Study the drawing (mm; zero at the part's minimum x, y, z) and answer. Round coordinates to 2 decimals unless told otherwise and drop trailing zeros. Loops run counter-clockwise (first coordinate to the right, second up) from the corner with the lowest first, then second, coordinate; pieces in that order, holes last. Notation, with made-up numbers: (88.5, 63) - (112.5, 63) arc R27 cw to (112.5, 89) - close; hole circle Ø3 at (35.25, -31.5). An arc over 180 degrees is marked (long way). One line per item, written item: value.
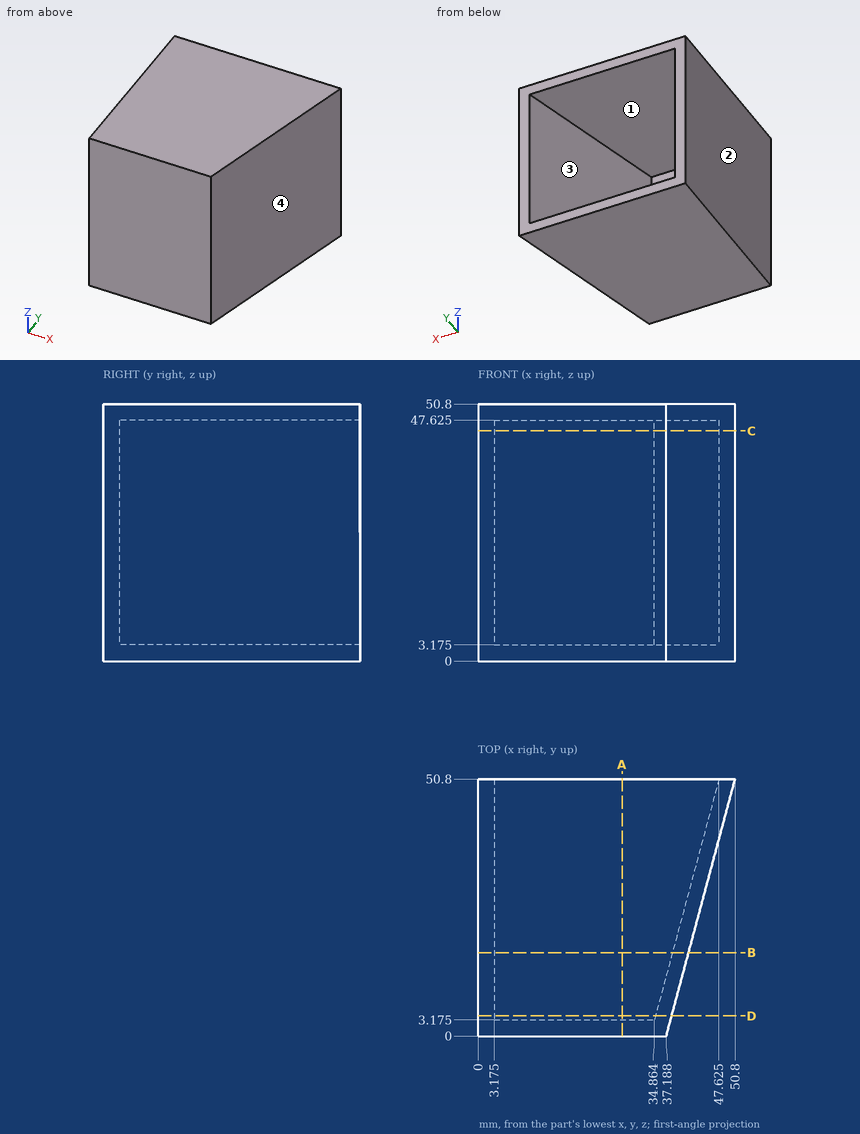
1) Consider L1, parallel to Z at x = 13.5, y = 14.5 (3 decimals); L2, parallel to Y at x = 8, z = 41.5 (3 decimals); L3, parallel to X at y = 43.5, z = 8.5 (1 decimal). Determine where each line is inside the solid, lowest interval first.
Final values:
L1: 0 to 3.175, 47.625 to 50.8
L2: 0 to 3.175
L3: 0 to 3.2, 45.7 to 48.8
2) A cutting plane is placed at A-A on x = 28.5. Give the vertices of the cut face in (y, z) (3 decimals).
Final values:
outline: (0, 0) - (50.8, 0) - (50.8, 3.175) - (3.175, 3.175) - (3.175, 47.625) - (50.8, 47.625) - (50.8, 50.8) - (0, 50.8) - close
3) A cutting plane is placed at D-D on y = 4. Give the vertices of the cut face in (x, z) (3 decimals).
Final values:
outline: (0, 0) - (38.26, 0) - (38.26, 50.8) - (0, 50.8) - close; hole (3.175, 3.175) - (35.085, 3.175) - (35.085, 47.625) - (3.175, 47.625) - close
4) A cutting plane is placed at B-B on y = 16.5. Give the vertices of the cut face in (x, z) (1 decimal).
Final values:
outline: (0, 0) - (41.6, 0) - (41.6, 50.8) - (0, 50.8) - close; hole (3.2, 3.2) - (38.4, 3.2) - (38.4, 47.6) - (3.2, 47.6) - close
5) For a pull along X with two mould halves and no side action, classify the marked faces 1, 2, 3 and 4 as released by +X, released by -X, zero draft, split by the parting line, or undercut.
Final values:
face 1: undercut
face 2: released by -X
face 3: undercut
face 4: released by +X
6) Each of these flat-tipped pins is pushed along its axis until it touches: pin 1 Ø22 at (y, z) = (30.5, 20.5) entering from +X; pin 2 Ø8 at (y, z) = (28, 12.5) entering from +X; pin 3 Ø2 at (x, z) = (7.5, 26.5) entering from +Y (3 decimals). Where does it stop, or does it pass through?
Final values:
pin 1: x = 48.31
pin 2: x = 45.76
pin 3: y = 3.175
7) A cutting plane is placed at C-C on z = 45.5. Give the vertices of the cut face in (x, y) (1 decimal).
Final values:
outline: (0, 0) - (37.2, 0) - (50.8, 50.8) - (47.6, 50.8) - (34.9, 3.2) - (3.2, 3.2) - (3.2, 50.8) - (0, 50.8) - close
